from build123d import *

# Parameters (mm, degrees)
EXTRUDE_THIN1_DEPTH = 5


with BuildPart() as part:
    # Sketch1 → Extrude-Thin1 (new, symmetric)
    with BuildSketch(Plane(origin=(0, 0, 0), x_dir=(1, 0, 0), z_dir=(0, 1, 0))):
        with BuildLine():
            Line((55.2, -36.678710461), (55.2, -16.678710461))
            ThreePointArc((55.2, -16.678710461), (0, 57.664715231), (-55.2, -16.678710461))
            Line((-55.2, -16.678710461), (-55.2, -36.678710461))
            Line((-55.2, -36.678710461), (-56.2, -36.678710461))
            Line((-56.2, -36.678710461), (-56.2, -16.825837665))
            ThreePointArc((-56.2, -16.825837665), (0, 58.664715231), (56.2, -16.825837665))
            Line((56.2, -16.825837665), (56.2, -36.678710461))
            Line((56.2, -36.678710461), (55.2, -36.678710461))
        make_face()
    extrude(amount=EXTRUDE_THIN1_DEPTH, both=True)


solid = part.part
Geometry check sheet. Reference: the model listing, model coordinates, mm. A direction names the side the tool comes from. Round coordinates to 2 decimals unless told otherwise and drop trailing zeros. Write each loop counter-clockwise with the first axis right and the second up, starting at its lowest first coordinate (ties: lowest second). Pieces come first, ordered by that corner, then holes. Notation, with made-up numbers: (42, -25.5) - (97, -25.5) arc R12 cw to (97, -21.5) - close; hole circle Ø4 at (41.5, 11). An arc over 180 degrees is marked (long way). One line per item, written item: value.
1. Scan lines: L1, parallel to X at y = 0.25, z = 0; L2, parallel to X at y = 4.25, z = 27; L3, parallel to Z at x = 0, y = 0.5. Record each from-to range of solid material in increasing order.
The answers:
L1: x = -58.66 to -57.66, 57.66 to 58.66
L2: x = -56.2 to -55.2, 55.2 to 56.2
L3: z = -58.66 to -57.66
2. Mould release check, pull along X, two halves, no side actions. Record for faces 6 (the face through (-1.529, 0.07, -58.645)), 7 (the face through (8.96, 5, -57.12)), 8 (the face through (-55.2, 0, 27)): released by +X, released by -X, zero draft, split by the parting line, or undercut.
The answers:
face 6: split by the parting line
face 7: zero draft
face 8: undercut
3. Cross-section at A-A on z = 0. Record the boundary of the cut face in (x, y).
The answers:
outline: (-58.66, -5) - (-57.66, -5) - (-57.66, 5) - (-58.66, 5) - close; (57.66, -5) - (58.66, -5) - (58.66, 5) - (57.66, 5) - close
4. Set-up check for faces 1 (the face through (8.96, -5, -57.12)), 2 (the face through (55.2, 0, 27)), 3 (the face through (-56.2, 0, 27)), 4 (the face through (56.2, 0, 27)), 5 (the face through (1.505, 0.07, -57.645)): record each of +Z, -Z, +X, -X, +Y, -Y from which the full face is reachable in a straight line by a thin tool's end or side.
The answers:
face 1: +Z, -Z, +X, -X, -Y
face 2: +Z, +Y, -Y
face 3: +Z, -X, +Y, -Y
face 4: +Z, +X, +Y, -Y
face 5: +Y, -Y
5. Cross-section at C-C on z = -13. Record the boundary of the cut face in (x, y).
The answers:
outline: (-57.21, -5) - (-56.18, -5) - (-56.18, 5) - (-57.21, 5) - close; (56.18, -5) - (57.21, -5) - (57.21, 5) - (56.18, 5) - close
6. Cross-section at B-B on y = 1. Record the boundary of the cut face in (x, z), and give its area (3 significant figures).
The answers:
outline: (-56.2, 16.83) arc R58.66 ccw (long way) to (56.2, 16.83) - (56.2, 36.68) - (55.2, 36.68) - (55.2, 16.68) arc R57.66 cw (long way) to (-55.2, 16.68) - (-55.2, 36.68) - (-56.2, 36.68) - close
area: 257 mm^2
7. Depth check by flat-ended pin: pin 1 Ø4 at (x, y) = (37.5, -0.5) entering from -Z; pin 2 Ø6 at (x, y) = (13.5, 0.5) entering from -Z; pin 3 Ø2 at (x, y) = (36.5, 1.5) entering from +Z. Enter the tip coordinate at first touch or a pass-through.
The answers:
pin 1: stops at z = -46.7
pin 2: stops at z = -57.72
pin 3: stops at z = -43.81
8. Cross-section at D-D on x = 0. Record the boundary of the cut face in (y, z), and give its area (3 significant figures).
The answers:
outline: (-5, -58.66) - (5, -58.66) - (5, -57.66) - (-5, -57.66) - close
area: 10.0 mm^2
